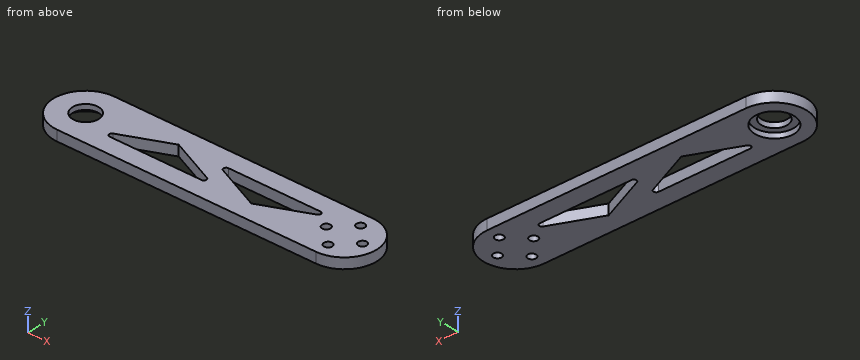
```python
from build123d import *

# Parameters (mm, degrees)
SKETCH_1_R          = 5
SKETCH_1_R_2        = 1.6
EXTRUDE_1_DEPTH     = 4
SKETCH_4_R          = 7.5
CUT_EXTRUDE_3_DEPTH = 3
CUT_EXTRUDE_4_REACH = 6


with BuildPart() as part:
    # 草图1 → 凸台-拉伸1 (new body)
    with BuildSketch(Plane.XY):
        with BuildLine():
            Line((0, 12.25), (100, 12.25))
            ThreePointArc((100, 12.25), (112.25, 0), (100, -12.25))
            Line((100, -12.25), (0, -12.25))
            ThreePointArc((0, -12.25), (-12.25, 0), (0, 12.25))
        make_face()
        Circle(SKETCH_1_R, mode=Mode.SUBTRACT)
        with Locations((100, 7)):
            Circle(SKETCH_1_R_2, mode=Mode.SUBTRACT)
        with Locations((107, 0)):
            Circle(SKETCH_1_R_2, mode=Mode.SUBTRACT)
        with Locations((100, -7)):
            Circle(SKETCH_1_R_2, mode=Mode.SUBTRACT)
        with Locations((93, 0)):
            Circle(SKETCH_1_R_2, mode=Mode.SUBTRACT)
    extrude(amount=EXTRUDE_1_DEPTH)

    # 草图4 → 切除-拉伸3 (cut)
    with BuildSketch(Plane.XY.offset(2)):
        Circle(SKETCH_4_R)
    extrude(amount=-CUT_EXTRUDE_3_DEPTH, mode=Mode.SUBTRACT)

    # 草图5 → 切除-拉伸4 (cut, up to next)
    with BuildSketch(Plane.XY.offset(4), mode=Mode.PRIVATE) as cut_extrude_4_sk1:
        with BuildLine():
            Line((31.5, 5), (13.306075984, -3.086188451))
            ThreePointArc((13.306075984, -3.086188451), (12.733998843, -4.207591488), (13.71221445, -5))
            Line((13.71221445, -5), (49.28778555, -5))
            ThreePointArc((49.28778555, -5), (50.266001157, -4.207591488), (49.693924016, -3.086188451))
            Line((49.693924016, -3.086188451), (31.5, 5))
        make_face()
    cut_extrude_4_tool1 = extrude(cut_extrude_4_sk1.sketch, amount=-CUT_EXTRUDE_4_REACH, mode=Mode.PRIVATE) & part.part
    add(cut_extrude_4_tool1.solids().sort_by_distance((31.5, -1.58127, 4))[0], mode=Mode.SUBTRACT)
    # 草图5 → 切除-拉伸4 (cut, up to next)
    with BuildSketch(Plane.XY.offset(4), mode=Mode.PRIVATE) as cut_extrude_4_sk2:
        with BuildLine():
            Line((68.5, -5), (86.693924016, 3.086188451))
            ThreePointArc((86.693924016, 3.086188451), (87.266001157, 4.207591488), (86.28778555, 5))
            Line((86.28778555, 5), (50.71221445, 5))
            ThreePointArc((50.71221445, 5), (49.733998843, 4.207591488), (50.306075984, 3.086188451))
            Line((50.306075984, 3.086188451), (68.5, -5))
        make_face()
    cut_extrude_4_tool2 = extrude(cut_extrude_4_sk2.sketch, amount=-CUT_EXTRUDE_4_REACH, mode=Mode.PRIVATE) & part.part
    add(cut_extrude_4_tool2.solids().sort_by_distance((68.5, 1.58127, 4))[0], mode=Mode.SUBTRACT)


solid = part.part
```
Could you check a few things on this model? Use its own coordinates, in mm. Coordinates: 2 decimals unless noted, no trailing zeros. Write each loop counter-clockwise with the first axis right and the second up, starting at its lowest first coordinate (ties: lowest second). Pieces come first, ordered by that corner, then holes. Notation, with made-up numbers: (-13.75, -13) -> (16.25, -13) arc R18 cw to (16.25, -9) -> close; hole circle Ø2 at (76.5, 43). An arc over 180 degrees is marked (long way). Write item = value, one per line. Start each with the question number.
(1) I want a section at C-C (x = 17.5). Please give me the cut outline in (y, z).
(2) I need wall thicknesses on line 1 (Y direction, x = 100, z = 2.2); line 2 (Y direction, x = 93, z = 2.65); line 3 (X direction, y = -5.75, z = 0.9). Which ranges of each line are inside material? Lowest first, please. Write a range as [from, to].
(3) I want a section at A-A (y = 0). Please give me the cut outline in (x, z), plus the area to 3 significant figures.
(4) I want a section at B-B (z = 1.05). Please give me the cut outline in (x, y).
(5) Will this pin go through, and if not, where does the flat tip stop? pin 1 (11.5 mm diameter, centred on x = 0, y = 0, fed in from -Z).
(6) I want a section at D-D (x = 93). Please give me the cut outline in (y, z), plus the area to 3 significant figures.
Result set:
q1.outline = (-12.25, 0) -> (-5, 0) -> (-5, 4) -> (-12.25, 4) -> close; (-1.22, 0) -> (12.25, 0) -> (12.25, 4) -> (-1.22, 4) -> close
q2.line_1 = [-12.25, -8.6], [-5.4, 5.4], [8.6, 12.25]
q2.line_2 = [-12.25, -1.6], [1.6, 12.25]
q2.line_3 = [-10.82, -4.82], [4.82, 99], [101, 110.82]
q3.outline = (-12.25, 0) -> (-7.5, 0) -> (-7.5, 2) -> (-5, 2) -> (-5, 4) -> (-12.25, 4) -> close; (5, 2) -> (7.5, 2) -> (7.5, 0) -> (20.25, 0) -> (20.25, 4) -> (5, 4) -> close; (42.75, 0) -> (57.25, 0) -> (57.25, 4) -> (42.75, 4) -> close; (79.75, 0) -> (91.4, 0) -> (91.4, 4) -> (79.75, 4) -> close; (94.6, 0) -> (105.4, 0) -> (105.4, 4) -> (94.6, 4) -> close; (108.6, 0) -> (112.25, 0) -> (112.25, 4) -> (108.6, 4) -> close
q3.area = 242 mm2
q4.outline = (0, -12.25) -> (100, -12.25) arc R12.25 ccw to (100, 12.25) -> (0, 12.25) arc R12.25 ccw to start; hole circle Ø15 at (0, 0); hole (13.31, -3.09) arc R1 ccw to (13.71, -5) -> (49.29, -5) arc R1 ccw to (49.69, -3.09) -> (31.5, 5) -> close; hole (50.31, 3.09) -> (68.5, -5) -> (86.69, 3.09) arc R1 ccw to (86.29, 5) -> (50.71, 5) arc R1 ccw to start; hole circle Ø3.2 at (93, 0); hole circle Ø3.2 at (100, -7); hole circle Ø3.2 at (100, 7); hole circle Ø3.2 at (107, 0)
q5.pin_1 = 2
q6.outline = (-12.25, 0) -> (-1.6, 0) -> (-1.6, 4) -> (-12.25, 4) -> close; (1.6, 0) -> (12.25, 0) -> (12.25, 4) -> (1.6, 4) -> close
q6.area = 85.2 mm2
